Drawing for the job (mm, zero at the part's lowest x, y, z). Coordinates: 2 decimals unless noted, no trailing zeros. Write each loop counter-clockwise with the first axis right and the second up, starting at its lowest first coordinate (ties: lowest second). Pieces come first, ordered by that corner, then holes. Notation, with made-up numbers: M 80,85 L 113,85 A28 ccw 113,105 Z; hole C 15,-9.5 d10. An arc over 180 degrees is marked long. Put each result on its own line as item: value. Start each with the question number.
Q1. Cut at A-A (z = 8). Write the cut outline in (x, y).
Q2. Cut at C-C (y = 1.75). Write the cut outline in (x, z), then the cut area to 3 significant figures.
Q3. Drill centre lines: line 1 along Z through (x, y) = (8, 10.5); line 2 along Y through (x, z) = (9.75, 1); line 3 along Z through (x, y) = (8, 4.25). Where is each one in solid material? Low to high.
Q4. Cut at B-B (x = 8). Write the cut outline in (y, z).
Q5. Pull direction Y, two halves, no side cores. Call the marked faces 1, 2, 3 and 4: pulls with the +Y half, pulls with the -Y half, needs draft (parallel to the pull), parting line crosses it, or undercut.
Q6. Cut at D-D (x = 14.75). Write the cut outline in (y, z), then the cut area to 3 significant figures.
Q7. Drop flat-ended pins along their axis: pin 1 (1 mm diameter, centred on x = 1.5, y = 7, fed in from +Z); pin 2 (1.5 mm diameter, centred on x = 9, z = 2, fed in from -Y); pin 3 (4.5 mm diameter, centred on x = 8, z = 8, fed in from -Y); pin 4 (2 mm diameter, centred on y = 11.5, z = 13, fed in from -X). Give the stop position or say it passes through.
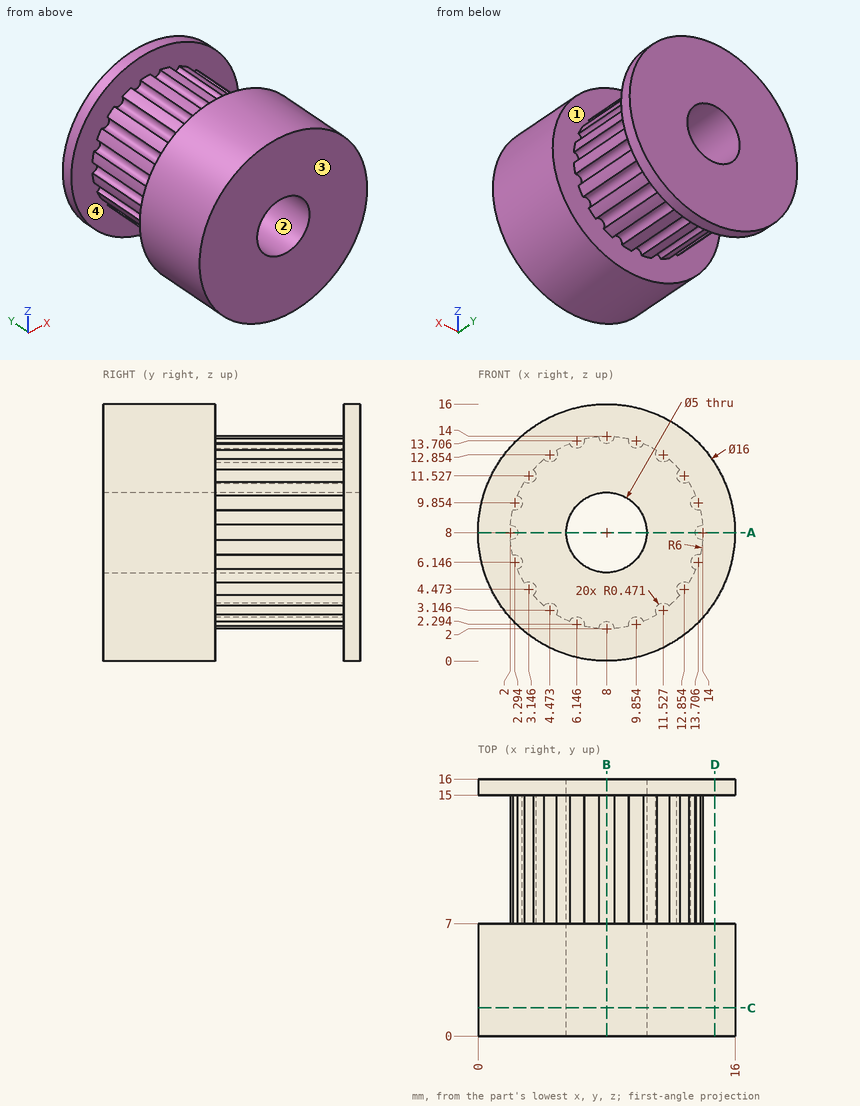
Computed values:
1. outline: M 0,0 L 5.5,0 L 5.5,16 L 0,16 L 0,15 L 2.47,15 L 2.47,7 L 0,7 Z; M 10.5,0 L 16,0 L 16,7 L 13.53,7 L 13.53,15 L 16,15 L 16,16 L 10.5,16 Z
2. outline: C 8,8 d16; hole C 8,8 d5
2. area: 181 mm2
3. line 1: 2.47 to 5.5, 10.5 to 13.53
3. line 2: 0 to 7, 15 to 16
3. line 3: 0 to 5.5, 10.5 to 16
4. outline: M 0,0 L 7,0 L 7,2.47 L 15,2.47 L 15,0 L 16,0 L 16,5.5 L 0,5.5 Z; M 0,10.5 L 16,10.5 L 16,16 L 15,16 L 15,13.53 L 7,13.53 L 7,16 L 0,16 Z
5. face 1: undercut
5. face 2: needs draft
5. face 3: pulls with the -Y half
5. face 4: undercut
6. outline: M 0,3.71 L 7,3.71 L 7,12.29 L 0,12.29 Z; M 15,3.71 L 16,3.71 L 16,12.29 L 15,12.29 Z
6. area: 68.7 mm2
7. pin 1: z = 13.29
7. pin 2: y = 0
7. pin 3: through
7. pin 4: x = 3.53
